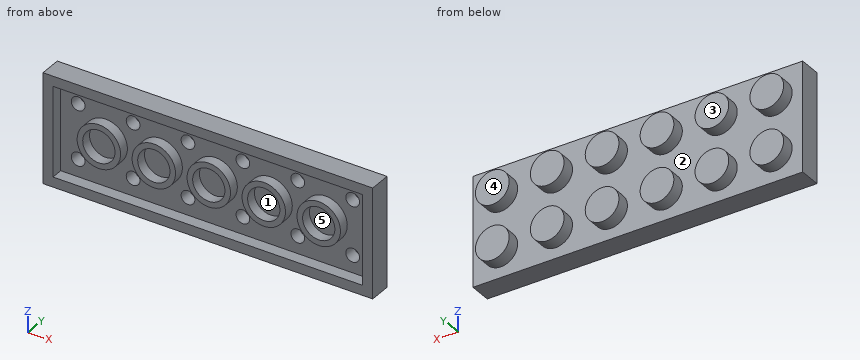
```python
from build123d import *

# Parameters (mm, degrees)
SKETCH2_W           = 47.81
SKETCH2_H           = 15.925
BOSS_EXTRUDE1_DEPTH = 3.16
SKETCH3_R           = 2.445
BOSS_EXTRUDE2_DEPTH = 1.88
SHELL1_T            = -1.45
SKETCH4_R           = 3.15
SKETCH4_R_2         = 2.34
BOSS_EXTRUDE3_DEPTH = 1.51


with BuildPart() as part:
    # Sketch2 → Boss-Extrude1 (new body)
    with BuildSketch(Plane(origin=(0, 0, 0), x_dir=(1, 0, 0), z_dir=(0, 1, 0))):
        Rectangle(SKETCH2_W, SKETCH2_H)
    extrude(amount=-BOSS_EXTRUDE1_DEPTH)

    # Sketch3 → Boss-Extrude2 (add)
    with BuildSketch(Plane(origin=(0, 0, 0), x_dir=(1, 0, 0), z_dir=(0, 1, 0))):
        with Locations(Location((-19.920833333, 3.98, 0), (0, 0, 270))):
            Circle(SKETCH3_R)
        with Locations(Location((-11.960833333, 3.98, 0), (0, 0, 270))):
            Circle(SKETCH3_R)
        with Locations(Location((-4.000833333, 3.98, 0), (0, 0, 270))):
            Circle(SKETCH3_R)
        with Locations(Location((3.959166667, 3.98, 0), (0, 0, 270))):
            Circle(SKETCH3_R)
        with Locations(Location((11.919166667, 3.98, 0), (0, 0, 270))):
            Circle(SKETCH3_R)
        with Locations(Location((19.879166667, 3.98, 0), (0, 0, 270))):
            Circle(SKETCH3_R)
        with Locations(Location((-11.960833333, -3.98, 0), (0, 0, 270))):
            Circle(SKETCH3_R)
        with Locations(Location((-4.000833333, -3.98, 0), (0, 0, 270))):
            Circle(SKETCH3_R)
        with Locations(Location((3.959166667, -3.98, 0), (0, 0, 270))):
            Circle(SKETCH3_R)
        with Locations(Location((11.919166667, -3.98, 0), (0, 0, 270))):
            Circle(SKETCH3_R)
        with Locations(Location((19.879166667, -3.98, 0), (0, 0, 270))):
            Circle(SKETCH3_R)
        with Locations(Location((-19.920833333, -3.98, 0), (0, 0, 270))):
            Circle(SKETCH3_R)
    extrude(amount=BOSS_EXTRUDE2_DEPTH)

    # Shell1
    shell1_openings = [part.faces().sort_by_distance(p)[0] for p in [
        (0, -3.16, 0),
    ]]
    offset(amount=SHELL1_T, openings=shell1_openings, kind=Kind.INTERSECTION)

    # Sketch4 → Boss-Extrude3 (add)
    # profile 1 of 5: a face of its own
    with BuildSketch(Plane.XZ.offset(1.45)):
        with Locations(Location((-15.936666667, 0.0025, 0), (0, 0, 90))):
            Circle(SKETCH4_R)
        with Locations(Location((-15.936666667, 0.0025, 0), (0, 0, 90))):
            Circle(SKETCH4_R_2, mode=Mode.SUBTRACT)
    # profile 2 of 5: a face of its own
    with BuildSketch(Plane.XZ.offset(1.45)):
        with Locations(Location((-7.966666667, 0.0025, 0), (0, 0, 90))):
            Circle(SKETCH4_R)
        with Locations(Location((-7.966666667, 0.0025, 0), (0, 0, 90))):
            Circle(SKETCH4_R_2, mode=Mode.SUBTRACT)
    # profile 3 of 5: a face of its own
    with BuildSketch(Plane.XZ.offset(1.45)):
        with Locations(Location((0.003333333, 0.0025, 0), (0, 0, 90))):
            Circle(SKETCH4_R)
        with Locations(Location((0.003333333, 0.0025, 0), (0, 0, 90))):
            Circle(SKETCH4_R_2, mode=Mode.SUBTRACT)
    # profile 4 of 5: a face of its own
    with BuildSketch(Plane.XZ.offset(1.45)):
        with Locations(Location((7.973333333, 0.0025, 0), (0, 0, 90))):
            Circle(SKETCH4_R)
        with Locations(Location((7.973333333, 0.0025, 0), (0, 0, 90))):
            Circle(SKETCH4_R_2, mode=Mode.SUBTRACT)
    # profile 5 of 5: a face of its own
    with BuildSketch(Plane.XZ.offset(1.45)):
        with Locations(Location((15.943333333, 0.0025, 0), (0, 0, 90))):
            Circle(SKETCH4_R)
        with Locations(Location((15.943333333, 0.0025, 0), (0, 0, 90))):
            Circle(SKETCH4_R_2, mode=Mode.SUBTRACT)
    extrude(amount=BOSS_EXTRUDE3_DEPTH)


solid = part.part
```
Source: CAD feature listing. Evaluate the final solid. Frame: model axes, mm. Face numbers are marked on the shaded views. A direction names the side the tool comes from. Round coordinates to 2 decimals unless told otherwise and drop trailing zeros. Write each loop counter-clockwise with the first axis right and the second up, starting at its lowest first coordinate (ties: lowest second). Pieces come first, ordered by that corner, then holes. Notation, with made-up numbers: M -15,-37.5 L -11,-37.5 A15 cw -11,-32.5 Z; hole C 12,68.5 d1. An arc over 180 degrees is marked long. Use CSV: the item, a comma, the result in double quotes. Start each with the question number.
Q1. Pull-direction query (Z, two-part tool) for the marked faces 4 and 5; classes: +Z half, -Z half, draft (parallel to the pull), parting line (faces both ways), or undercut.
Q2. Cut plane C-C on x = -9. Output: boundary loops of the cut face in (y, z).
Q3. Cut plane A-A on y = -2.1. Count the separate pieces of the cut face and the enclosed holes in it, plus the area to 3 significant figures.
Q4. First-contact query: P1, Ø7.5, axis at x = 0, z = 0, coming from the -Y side; P2, Ø1.2, axis at x = 19.88, z = -3.98, coming from the -Y side; P3, Ø1.6, axis at x = 19.5, z = -4, coming from the -Y side. Flat tips, straight axial feed; report the tip coordinate or a pass-through.
Q5. Line query: line 1 (Z direction, x = 16, y = -2.1); line 2 (X direction, y = 1.35, z = -3.5); line 3 (X direction, y = 0.95, z = -3). Output: solid intervals per line, ascending. Write a range as from..to.
Q6. Access query for the marked faces 1, 2 and 3. Directions: +Z, -Z, +X, -X, +Y, -Y. A direction counts if a zero-diameter tool reaches every point of the face in a straight line with its end or side. Return the directions, or none.
Results found:
1,face 4,"draft"
1,face 5,"undercut"
2,outline,"M -3.16,-7.96 L 0,-7.96 L 0,7.96 L -3.16,7.96 L -3.16,6.51 L -1.45,6.51 L -1.45,2.98 L -2.96,2.98 L -2.96,2.1 L -1.45,2.1 L -1.45,-2.1 L -2.96,-2.1 L -2.96,-2.97 L -1.45,-2.97 L -1.45,-6.51 L -3.16,-6.51 Z"
3,separate pieces,"6"
3,enclosed holes,"6"
3,area,"246 mm^2"
4,P1,"y = -2.96"
4,P2,"y = 0.43"
4,P3,"y = -1.45"
5,line 1,"-7.96..-6.51, -3.15..-2.34, 2.34..3.15, 6.51..7.96"
5,line 2,"-22.32..-17.52, -14.36..-9.56, -6.4..-1.6, 1.56..6.36, 9.52..14.32, 17.48..22.28"
5,line 3,"-22.16..-17.68, -14.2..-9.72, -6.24..-1.76, 1.72..6.2, 9.68..14.16, 17.64..22.12"
6,face 1,"-Y"
6,face 2,"+Y"
6,face 3,"+Z, -Z, +X, -X, +Y"
